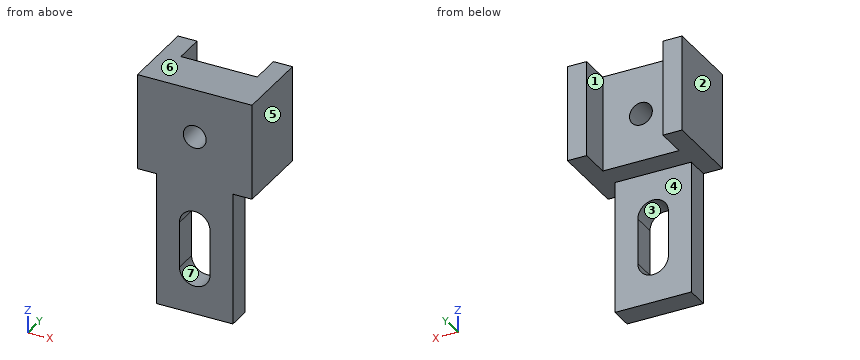
Autodesk Fusion 360 part; units mm, degrees
sketch "Sketch1" plane through (0, 0, 0) normal (0, 1, 0) x (1, 0, 0) in component "Slider"
  line L0 (9.525, 8) -> (-9.525, 8)
  line L1 (9.525, -8) -> (9.525, 8)
  line L2 (-9.525, -8) -> (9.525, -8)
  line L3 (-9.525, 8) -> (-9.525, -8)
  line L4 (-6.35, 30.1) -> (-6.35, -8)
  line L5 (6.35, 30.1) -> (-6.35, 30.1)
  line L6 (6.35, -8) -> (6.35, 30.1)
  line L7 (-2.54, 22.86) -> (-2.54, 15.24)
  arc A0 (-2.54, 15.24) -> (2.54, 15.24) centre (0, 15.24) ccw
  line L8 (2.54, 15.24) -> (2.54, 22.86)
  arc A1 (2.54, 22.86) -> (-2.54, 22.86) centre (0, 22.86) ccw
  line L9 (0, 25.4) -> (0, 12.7) construction
  circle A2 centre (0, 0) radius 1.8987
  circle A3 centre (0, 0) radius 3.175
  circle A4 centre (0, 0) radius 12.7 construction
  circle A5 centre (0, 15.24) radius 3.9624 construction
  circle A6 centre (0, 22.86) radius 3.9624 construction
  point P0 (0, 0)
  dimension "d2_1" = 5.08
  dimension "d4_1" = 6.35
  dimension "d5_1" = 3.7973
  dimension "d9_1" = 19.05
  dimension "d10_1" = 6.35
  dimension "d12_1" = 6.35
  dimension "d15_1" = 15.24
  dimension "d16_1" = 12.7
  dimension "d19_1" = 9.525
  dimension "d50_1" = 8
  dimension "d51_1" = 8
  dimension "d52_1" = 25.4
  dimension "d53_1" = 7.9248
  dimension "d54_1" = 7.9248
  dimension "d55_1" = 38.1
extrude "Extrude1" add sketch "Sketch1" along normal blind 3.81 contours L0 L2 L4 L6 | L0 L4 L5 L6 in component "Slider"
extrude "Extrude2" add sketch "Sketch1" along normal blind 7.62 contours L0 L2 L4 L6 | A3 in component "Slider"
extrude "Extrude3" add sketch "Sketch1" along normal blind 12.7 contours L0 L1 L2 L6 | L0 L2 L3 L4 in component "Slider"
thread "Thread1" in component "Slider"
component "Slider" placed x (1, 0, 0) y (0, 1, 0) z (0, 0, 1) at (0, 0, 0)
equation "d12_1 = d10_1"
equation "d53_1 = ( 3.9624 * 2 ) * 1 mm"
equation "d54_1 = d53_1"
Build history of the part. All positions in model axes, mm. Face numbers are marked on the shaded views. A direction names the side the tool comes from. Coordinates: 2 decimals unless noted, no trailing zeros. Order: outer loops, then holes, each group sorted by start corner. A loop starts at its lowest first (then second) coordinate and runs counter-clockwise, first axis right, second up. Notation, with made-up numbers: (79, -23.75) -> (128, -23.75) arc R24 ccw to (128, -5.75) -> close; hole circle Ø6 at (40.25, 19). An arc over 180 degrees is marked (long way). One line per item, written item: value.
(1) Drop flat-ended pins along their axis: pin 1 Ø3 at (x, z) = (2, -4.5) entering from -Y; pin 2 Ø1.9 at (y, z) = (2.5, -19) entering from -X; pin 3 Ø5 at (x, z) = (0, 0) entering from +Y; pin 4 Ø4 at (y, z) = (1.5, -19.5) entering from +X. Give the stop position or say it passes through.
Checked values:
pin 1: y = 0
pin 2: x = -6.35
pin 3: y = 7.62
pin 4: x = 6.35
(2) Mould opens along Z. For the marked faces 5, 6 and 7 say: pulls with the +Z half, pulls with the -Z half, needs draft (parallel to the pull), parting line crosses it, or undercut.
Checked values:
face 5: needs draft
face 6: pulls with the +Z half
face 7: undercut
(3) Slice it at C-C, the plane y = 10.75. List the corners of the cut face in (x, z) (3 decimals), plus the area to 3 significant figures.
Checked values:
outline: (-9.525, -8) -> (-6.35, -8) -> (-6.35, 8) -> (-9.525, 8) -> close; (6.35, -8) -> (9.525, -8) -> (9.525, 8) -> (6.35, 8) -> close
area: 102 mm2
(4) Tool access for the marked faces 1, 2, 3 and 4: list every direction of +Z, -Z, +X, -X, +Y, -Y with a clear straight run to the whole face (end or side of a thin tool).
Checked values:
face 1: +Z, -Z, +Y
face 2: +Z, -Z, -X, +Y, -Y
face 3: +Y, -Y
face 4: -Z, +X, -X, +Y
(5) Slice it at A-A, the plane z = 0. List the corners of the cut face in (x, y) (3 decimals), plus the area to 3 significant figures.
Checked values:
outline: (-9.525, 0) -> (-1.899, 0) -> (-1.899, 7.62) -> (-6.35, 7.62) -> (-6.35, 12.7) -> (-9.525, 12.7) -> close; (1.899, 0) -> (9.525, 0) -> (9.525, 12.7) -> (6.35, 12.7) -> (6.35, 7.62) -> (1.899, 7.62) -> close
area: 148 mm2
(6) Slice it at D-D, the plane y = 1.5. List the corners of the cut face in (x, z) (3 decimals).
Checked values:
outline: (-9.525, -8) -> (-6.35, -8) -> (-6.35, -30.1) -> (6.35, -30.1) -> (6.35, -8) -> (9.525, -8) -> (9.525, 8) -> (-9.525, 8) -> close; hole (-2.54, -22.86) arc R2.54 ccw to (2.54, -22.86) -> (2.54, -15.24) arc R2.54 ccw to (-2.54, -15.24) -> close; hole circle Ø3.797 at (0, 0)
(7) Probe line 1 (Z direction, x = 0, y = 2.5); line 2 (X direction, y = 2.25, z = 0) (3 decimals); line 3 (Z direction, x = 0, y = 4). List the from-to ranges inside material, lowest first. Write a range as [from, to].
Checked values:
line 1: [-30.1, -25.4], [-12.7, -1.9], [1.9, 8]
line 2: [-9.525, -1.899], [1.899, 9.525]
line 3: [-8, -1.9], [1.9, 8]
(8) Slice it at B-B, the plane x = 0. List the corners of the cut face in (y, z).
Checked values:
outline: (0, -30.1) -> (3.81, -30.1) -> (3.81, -25.4) -> (0, -25.4) -> close; (0, -12.7) -> (3.81, -12.7) -> (3.81, -8) -> (7.62, -8) -> (7.62, -1.9) -> (0, -1.9) -> close; (0, 1.9) -> (7.62, 1.9) -> (7.62, 8) -> (0, 8) -> close
